Read the model definition and answer for the solid it produces. Units are mm, in the model's axes. Face numbers are marked on the shaded views. A direction names the side the tool comes from. Coordinates: 2 decimals unless noted, no trailing zeros. Write each loop counter-clockwise with the first axis right and the second up, starting at its lowest first coordinate (ties: lowest second). Pieces come first, ordered by that corner, then holes. Notation, with made-up numbers: (25.25, 52.5) -> (66.25, 52.5) arc R21 ccw to (66.25, 84.5) -> close; hole circle Ø6 at (0, 74). An arc over 180 degrees is marked (long way). Return JSON: item names as keys, results as strings.
from build123d import *

# Parameters (mm, degrees)
MODEL_R             = 19.8387
BOSS_EXTRUDE1_DEPTH = 6.35


with BuildPart() as part:
    # Model → Boss-Extrude1 (new body)
    with BuildSketch(Plane.XY):
        Polygon((-20.5954, 132.4124), (-26.7451, 132.4124), (-26.7451, 151.262), (-84.9649, 151.262), (-84.9649, 132.4124), (-91.1147, 132.4124), (-91.1147, 107.2136), (-84.9649, 107.2136), (-84.9649, 81.2129), (-91.1147, 81.2129), (-91.1147, 56.0124), (-84.9649, 56.0124), (-84.9649, 37.1628), (-26.7451, 37.1628), (-26.7451, 56.0124), (-20.5954, 56.0124), (-20.5954, 81.2129), (-26.7451, 81.2129), (-26.7451, 107.2136), (-20.5954, 107.2136), align=None)
        with Locations((-55.8552, 94.2124)):
            Circle(MODEL_R, mode=Mode.SUBTRACT)
        with BuildLine():
            Line((-76.6319, 70.2547), (-78.6976, 68.1899))
            add(Edge.make_bspline(
                [(-78.6976, 68.1899), (-79.578, 67.3086), (-80.9971, 67.3086), (-81.878, 68.1903)],
                knots=[0.142857143, 0.142857143, 0.142857143, 0.142857143, 0.285714286, 0.285714286, 0.285714286, 0.285714286], degree=3))
            add(Edge.make_bspline(
                [(-81.878, 68.1903), (-82.7596, 69.0707), (-82.7601, 70.4902), (-81.878, 71.3707)],
                knots=[0.285714286, 0.285714286, 0.285714286, 0.285714286, 0.428571429, 0.428571429, 0.428571429, 0.428571429], degree=3))
            Line((-81.878, 71.3707), (-79.8123, 73.4364))
            add(Edge.make_bspline(
                [(-79.8123, 73.4364), (-78.9314, 74.3172), (-77.5119, 74.3172), (-76.6315, 73.4364)],
                knots=[0.571428571, 0.571428571, 0.571428571, 0.571428571, 0.714285714, 0.714285714, 0.714285714, 0.714285714], degree=3))
            add(Edge.make_bspline(
                [(-76.6315, 73.4364), (-75.7498, 72.5547), (-75.7498, 71.1368), (-76.6319, 70.2547)],
                knots=[0.714285714, 0.714285714, 0.714285714, 0.714285714, 1, 1, 1, 1], degree=3))
        make_face(mode=Mode.SUBTRACT)
        with BuildLine():
            Line((-29.8321, 117.0554), (-31.897, 114.9897))
            add(Edge.make_bspline(
                [(-31.897, 114.9897), (-32.7791, 114.1076), (-34.1965, 114.1076), (-35.0782, 114.9897)],
                knots=[0.142857143, 0.142857143, 0.142857143, 0.142857143, 0.285714286, 0.285714286, 0.285714286, 0.285714286], degree=3))
            add(Edge.make_bspline(
                [(-35.0782, 114.9897), (-35.959, 115.8705), (-35.959, 117.2896), (-35.0782, 118.1705)],
                knots=[0.285714286, 0.285714286, 0.285714286, 0.285714286, 0.428571429, 0.428571429, 0.428571429, 0.428571429], degree=3))
            Line((-35.0782, 118.1705), (-33.0129, 120.2357))
            add(Edge.make_bspline(
                [(-33.0129, 120.2357), (-32.1324, 121.1178), (-30.7129, 121.1178), (-29.8321, 120.2357)],
                knots=[0.571428571, 0.571428571, 0.571428571, 0.571428571, 0.714285714, 0.714285714, 0.714285714, 0.714285714], degree=3))
            add(Edge.make_bspline(
                [(-29.8321, 120.2357), (-28.95, 119.3553), (-28.9504, 117.9362), (-29.8321, 117.0554)],
                knots=[0.714285714, 0.714285714, 0.714285714, 0.714285714, 1, 1, 1, 1], degree=3))
        make_face(mode=Mode.SUBTRACT)
        with BuildLine():
            Line((-29.8321, 71.3707), (-31.8965, 73.4364))
            add(Edge.make_bspline(
                [(-31.8965, 73.4364), (-32.7786, 74.3172), (-34.1969, 74.3172), (-35.0786, 73.4364)],
                knots=[0.142857143, 0.142857143, 0.142857143, 0.142857143, 0.285714286, 0.285714286, 0.285714286, 0.285714286], degree=3))
            add(Edge.make_bspline(
                [(-35.0786, 73.4364), (-35.959, 72.5547), (-35.959, 71.1364), (-35.0786, 70.2543)],
                knots=[0.285714286, 0.285714286, 0.285714286, 0.285714286, 0.428571429, 0.428571429, 0.428571429, 0.428571429], degree=3))
            Line((-35.0786, 70.2543), (-33.0129, 68.1899))
            add(Edge.make_bspline(
                [(-33.0129, 68.1899), (-32.1324, 67.3082), (-30.7129, 67.3086), (-29.8325, 68.1903)],
                knots=[0.571428571, 0.571428571, 0.571428571, 0.571428571, 0.714285714, 0.714285714, 0.714285714, 0.714285714], degree=3))
            add(Edge.make_bspline(
                [(-29.8325, 68.1903), (-28.9504, 69.0707), (-28.95, 70.4902), (-29.8321, 71.3707)],
                knots=[0.714285714, 0.714285714, 0.714285714, 0.714285714, 1, 1, 1, 1], degree=3))
        make_face(mode=Mode.SUBTRACT)
        with BuildLine():
            Line((-76.6319, 118.1705), (-78.6976, 120.2357))
            add(Edge.make_bspline(
                [(-78.6976, 120.2357), (-79.578, 121.1178), (-80.9975, 121.1178), (-81.878, 120.2357)],
                knots=[0.142857143, 0.142857143, 0.142857143, 0.142857143, 0.285714286, 0.285714286, 0.285714286, 0.285714286], degree=3))
            add(Edge.make_bspline(
                [(-81.878, 120.2357), (-82.7601, 119.3553), (-82.7601, 117.9358), (-81.878, 117.0554)],
                knots=[0.285714286, 0.285714286, 0.285714286, 0.285714286, 0.428571429, 0.428571429, 0.428571429, 0.428571429], degree=3))
            Line((-81.878, 117.0554), (-79.8127, 114.9897))
            add(Edge.make_bspline(
                [(-79.8127, 114.9897), (-78.9322, 114.1076), (-77.5123, 114.1076), (-76.6319, 114.9897)],
                knots=[0.571428571, 0.571428571, 0.571428571, 0.571428571, 0.714285714, 0.714285714, 0.714285714, 0.714285714], degree=3))
            add(Edge.make_bspline(
                [(-76.6319, 114.9897), (-75.7498, 115.8705), (-75.7498, 117.29), (-76.6319, 118.1705)],
                knots=[0.714285714, 0.714285714, 0.714285714, 0.714285714, 1, 1, 1, 1], degree=3))
        make_face(mode=Mode.SUBTRACT)
        with BuildLine():
            add(Edge.make_bspline(
                [(-61.8264, 129.7262), (-60.4231, 129.7262), (-59.2852, 130.8633), (-59.2852, 132.2662)],
                knots=[0, 0, 0, 0, 0.2, 0.2, 0.2, 0.2], degree=3))
            add(Edge.make_bspline(
                [(-59.2852, 132.2662), (-59.2852, 133.6691), (-60.4231, 134.8074), (-61.8264, 134.8074)],
                knots=[0.2, 0.2, 0.2, 0.2, 0.4, 0.4, 0.4, 0.4], degree=3))
            add(Edge.make_bspline(
                [(-61.8264, 134.8074), (-63.2289, 134.8074), (-64.366, 133.6691), (-64.366, 132.2662)],
                knots=[0.4, 0.4, 0.4, 0.4, 0.6, 0.6, 0.6, 0.6], degree=3))
            add(Edge.make_bspline(
                [(-64.366, 132.2662), (-64.366, 130.8633), (-63.2289, 129.7262), (-61.8264, 129.7262)],
                knots=[0.6, 0.6, 0.6, 0.6, 1, 1, 1, 1], degree=3))
        make_face(mode=Mode.SUBTRACT)
        with BuildLine():
            add(Edge.make_bspline(
                [(-61.8264, 53.5264), (-60.4231, 53.5264), (-59.2852, 54.6635), (-59.2852, 56.0664)],
                knots=[0, 0, 0, 0, 0.2, 0.2, 0.2, 0.2], degree=3))
            add(Edge.make_bspline(
                [(-59.2852, 56.0664), (-59.2852, 57.4693), (-60.4231, 58.6076), (-61.8264, 58.6076)],
                knots=[0.2, 0.2, 0.2, 0.2, 0.4, 0.4, 0.4, 0.4], degree=3))
            add(Edge.make_bspline(
                [(-61.8264, 58.6076), (-63.2289, 58.6076), (-64.366, 57.4693), (-64.366, 56.0664)],
                knots=[0.4, 0.4, 0.4, 0.4, 0.6, 0.6, 0.6, 0.6], degree=3))
            add(Edge.make_bspline(
                [(-64.366, 56.0664), (-64.366, 54.6635), (-63.2289, 53.5264), (-61.8264, 53.5264)],
                knots=[0.6, 0.6, 0.6, 0.6, 1, 1, 1, 1], degree=3))
        make_face(mode=Mode.SUBTRACT)
        with BuildLine():
            add(Edge.make_bspline(
                [(-49.884, 129.7262), (-48.4812, 129.7262), (-47.3445, 130.8633), (-47.3445, 132.2662)],
                knots=[0, 0, 0, 0, 0.2, 0.2, 0.2, 0.2], degree=3))
            add(Edge.make_bspline(
                [(-47.3445, 132.2662), (-47.3445, 133.6691), (-48.4812, 134.8074), (-49.884, 134.8074)],
                knots=[0.2, 0.2, 0.2, 0.2, 0.4, 0.4, 0.4, 0.4], degree=3))
            add(Edge.make_bspline(
                [(-49.884, 134.8074), (-51.2869, 134.8074), (-52.424, 133.6691), (-52.424, 132.2662)],
                knots=[0.4, 0.4, 0.4, 0.4, 0.6, 0.6, 0.6, 0.6], degree=3))
            add(Edge.make_bspline(
                [(-52.424, 132.2662), (-52.424, 130.8633), (-51.2869, 129.7262), (-49.884, 129.7262)],
                knots=[0.6, 0.6, 0.6, 0.6, 1, 1, 1, 1], degree=3))
        make_face(mode=Mode.SUBTRACT)
        with BuildLine():
            add(Edge.make_bspline(
                [(-49.884, 53.5264), (-48.4812, 53.5264), (-47.3445, 54.6635), (-47.3445, 56.0664)],
                knots=[0, 0, 0, 0, 0.2, 0.2, 0.2, 0.2], degree=3))
            add(Edge.make_bspline(
                [(-47.3445, 56.0664), (-47.3445, 57.4693), (-48.4812, 58.6076), (-49.884, 58.6076)],
                knots=[0.2, 0.2, 0.2, 0.2, 0.4, 0.4, 0.4, 0.4], degree=3))
            add(Edge.make_bspline(
                [(-49.884, 58.6076), (-51.2869, 58.6076), (-52.424, 57.4693), (-52.424, 56.0664)],
                knots=[0.4, 0.4, 0.4, 0.4, 0.6, 0.6, 0.6, 0.6], degree=3))
            add(Edge.make_bspline(
                [(-52.424, 56.0664), (-52.424, 54.6635), (-51.2869, 53.5264), (-49.884, 53.5264)],
                knots=[0.6, 0.6, 0.6, 0.6, 1, 1, 1, 1], degree=3))
        make_face(mode=Mode.SUBTRACT)
    extrude(amount=BOSS_EXTRUDE1_DEPTH)


solid = part.part
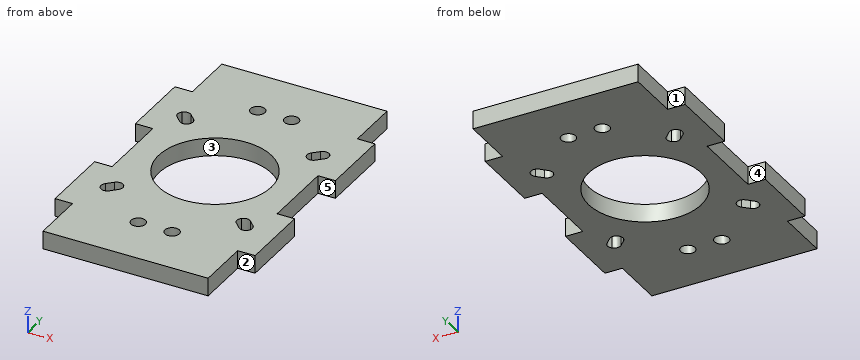
1. The part is cut by section A-A (y = 93). Determine the outline of the cut face in (x, z).
Taken from the geometry:
{"outline": "(-84.96, 0) -> (-75.66, 0) -> (-75.66, 6.35) -> (-84.96, 6.35) -> close; (-36.05, 0) -> (-26.75, 0) -> (-26.75, 6.35) -> (-36.05, 6.35) -> close"}
2. Flat-ended cylindrical pins translate along their axes: pin 1 Ø3 at (y, z) = (88.5, 3.5) entering from +X; pin 2 Ø1.9 at (y, z) = (49.5, 3) entering from -X; pin 3 Ø3 at (x, z) = (-22.5, 2) entering from -Y. Find the tip coordinate at first contact, or state that the pin passes through.
Taken from the geometry:
{"pin 1": "stops at x = -26.75", "pin 2": "stops at x = -84.96", "pin 3": "stops at y = 56.01"}
3. The part is cut by section C-C (z = 2.5). Count the separate pieces of the cut face and the enclosed holes in it, then the cut area to 3 significant figures.
Taken from the geometry:
{"separate pieces": "1", "enclosed holes": "9", "area": "5,830 mm2"}
4. The part is cut by section B-B (x = -73.5). Determine the outline of the cut face in (y, z).
Taken from the geometry:
{"outline": "(37.16, 0) -> (85.14, 0) -> (85.14, 6.35) -> (37.16, 6.35) -> close; (103.28, 0) -> (151.26, 0) -> (151.26, 6.35) -> (103.28, 6.35) -> close"}
5. A tool of negligible diameter and unlimited length cuts with its end or side. For the marked faces 1, 2, 3, 4 and 5, from which of +Z, -Z, +X, -X, +Y, -Y can it reach the whole face along a straight path? Write none if from no direction.
Taken from the geometry:
{"face 1": "+Z, -Z, -X, +Y", "face 2": "+Z, -Z, +X, -Y", "face 3": "+Z, -Z", "face 4": "+Z, -Z, -X", "face 5": "+Z, -Z, +X"}
6. Consider L1, parallel to Y at x = -55, z = 4.75; L2, parallel to Y at x = -24.5, z = 0.75; L3, parallel to X at y = 145.5, z = 5.25. Determine where each line is inside the solid, lowest interval first.
Taken from the geometry:
{"L1": "y = 37.16 to 74.39, 114.03 to 151.26", "L2": "y = 56.01 to 81.21, 107.21 to 132.41", "L3": "x = -84.96 to -26.75"}
